Can you work these out from the drawing? Everything is in mm from the part's minimum corner. Give positions to 0.01 mm unless a question says otherwise; leave off trailing zeros. Write each loop counter-clockwise with the first axis right and the second up, starting at its lowest first coordinate (ties: lowest second). Pieces come first, ordered by that corner, then holes. Notation, with made-up numbers: (-15, -30.75) -> (44, -30.75) arc R26 ccw to (44, -12.75) -> close; hole circle Ø5 at (64, 68). An arc over 180 degrees is marked (long way). Return JSON: item names as keys, results as strings.
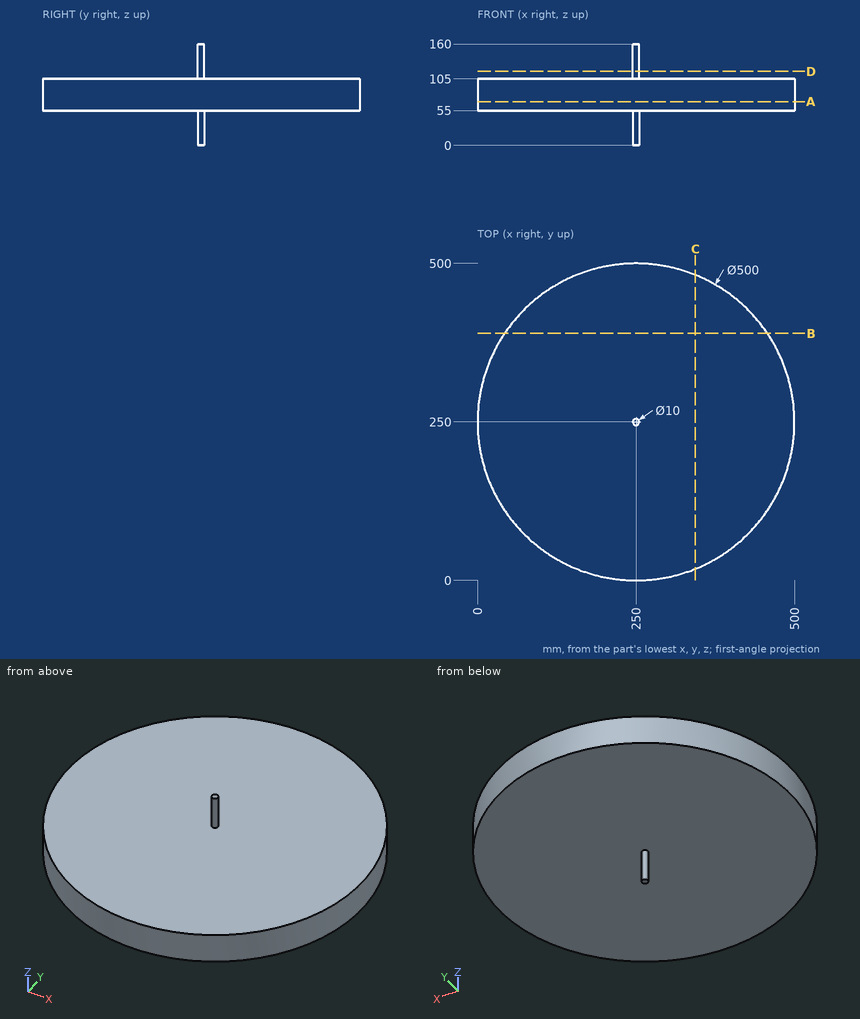
1. Suppose I cut it at D-D, the plane z = 117. List the corners of the cut face in (x, y) for me, and give its area (3 significant figures).
Taken from the geometry:
{"outline": "circle Ø10 at (250, 250)", "area": "78.5 mm²"}
2. For pin 1 Ø1 at (y, z) = (386.5, 101) entering from -X; pin 2 Ø8 at (x, y) = (75, 279) entering from -Z; pin 3 Ø2 at (x, z) = (189, 58) entering from +Y, each with a flat end and sliding along its axis, tell me the tip position at first contact or that it passes through.
Taken from the geometry:
{"pin 1": "stops at x = 40.23", "pin 2": "stops at z = 55", "pin 3": "stops at y = 492.69"}
3. Suppose I cut it at A-A, the plane z = 69. List the corners of the cut face in (x, y) for me, and give its area (3 significant figures).
Taken from the geometry:
{"outline": "circle Ø500 at (250, 250)", "area": "196,000 mm²"}
4. Suppose I cut it at C-C, the plane x = 343.5. List the corners of the cut face in (y, z) for me, and give its area (3 significant figures).
Taken from the geometry:
{"outline": "(18.14, 55) -> (481.86, 55) -> (481.86, 105) -> (18.14, 105) -> close", "area": "23,200 mm²"}
5. If I drill on line 1 (Z direction, x = 179.5, y = 479); line 2 (X direction, y = 251, z = 153.5); line 3 (X direction, y = 466, z = 64), over which ranges is the centre line in solid material (lowest first)? Write a range as [from, to].
Taken from the geometry:
{"line 1": "z = [55, 105]", "line 2": "x = [245.1, 254.9]", "line 3": "x = [124.13, 375.87]"}
6. Suppose I cut it at B-B, the plane y = 389.5. List the corners of the cut face in (x, z) for me, and give its area (3 significant figures).
Taken from the geometry:
{"outline": "(42.54, 55) -> (457.46, 55) -> (457.46, 105) -> (42.54, 105) -> close", "area": "20,700 mm²"}
